Source: CAD feature listing. Evaluate the final solid. Frame: model axes, mm. A direction names the side the tool comes from. Coordinates: 2 decimals unless noted, no trailing zeros. Order: outer loops, then holes, each group sorted by start corner. A loop starts at its lowest first (then second) coordinate and runs counter-clockwise, first axis right, second up. Notation, with made-up numbers: (-39.5, 9.25) -> (-33.5, 9.25) arc R26 ccw to (-33.5, 38.25) -> close; hole circle Ø10 at (-40, 72.25). An arc over 180 degrees is marked (long way). Write item = value, one per line. Start each with the question number.
Item 1: Contact query for flat-ended pins moving along their axis: pin 1 (3.5 mm diameter, centred on x = 35, y = -50, fed in from +Z); pin 2 (1.9 mm diameter, centred on x = 50, y = 5, fed in from -Z). Output: stop coordinate, or through.
Item 2: Section query C-C (y = 0). Output: boundary loops of the cut face in (x, z).
Item 3: Section query A-A (y = -45). Output: boundary loops of the cut face in (x, z).
Item 4: Set-up query: faces 1 (the cylindrical face through (-51.526, 50.481, -6.549)), 2 (the cylindrical face through (-33.5, 27.117, -1.479)), 3 (the cylindrical face through (3.35, 47.85, -4.93)). Return all of +Z, -Z, +X, -X, +Y, -Y with unobstructed straight access to the full face (end or side cutting, diameter ignored); none if empty.
Item 5: Ray query, line 1 along Y through (x, z) = (35, -7.25); line 2 along X through (y, z) = (-4.5, -2); line 3 along X through (y, z) = (-44, -5.75). Return the intervals inside material, ascending. Write a range as [from, to].
Item 6: Section query D-D (x = 0.5). Output: boundary loops of the cut face in (y, z), then the cut area to 3 significant figures.
Item 7: Section query B-B (x = 45). Output: boundary loops of the cut face in (y, z).
```python
from build123d import *

# Parameters (mm, degrees)
F0_W           = 110
F0_H           = 110
F1_DEPTH       = 10
F2_D           = 3.2
F2_CBORE_D     = 6.5
F2_CBORE_DEPTH = 3
F3_D           = 4.2
F6_D           = 3.3
F6_DEPTH       = 14.1
F6_TIP         = 0.9914200214
F6_ON_F4_D     = 3.3
F6_ON_F4_DEPTH = 14.1
F6_ON_F4_TIP   = 0.9914200214
F7_D           = 5


with BuildPart() as f1:
    # F0 (on Top) → F1 (new body)
    with BuildSketch(Plane.XY):
        Rectangle(F0_W, F0_H)
    extrude(amount=-F1_DEPTH)

    # F2 (through all)
    with Locations(Plane.XY):
        with Locations((-50, 30), (-35, 30), (-35, 50), (-50, 50), (-50, -30), (-35, -30), (-35, -50), (-50, -50), (35, -30), (35, -50), (50, -50), (50, -30), (35, 30), (35, 50), (50, 50), (50, 30), (-50, 5), (-50, -5), (50, 5), (50, -5)):
            CounterBoreHole(F2_D / 2, F2_CBORE_D / 2, F2_CBORE_DEPTH)

    # F3 (through all)
    with Locations(Plane.XY):
        with Locations((-45, 45), (45, 45), (45, -45), (-45, -45)):
            Hole(F3_D / 2)

    # F6
    with Locations(Plane(origin=(0, 55, 0), x_dir=(-1, 0, 0), z_dir=(0, 1, 0))):
        with Locations((-5, -5), (5, -5)):
            Hole(F6_D / 2, depth=F6_DEPTH)
            with Locations((0, 0, -(F6_DEPTH + F6_TIP / 2))):  # 118° drill point
                Cone(0, F6_D / 2, F6_TIP, mode=Mode.SUBTRACT)

    # F6 on F4
    with Locations(Plane.XZ.offset(55)):
        with Locations((-5, -5), (5, -5)):
            Hole(F6_ON_F4_D / 2, depth=F6_ON_F4_DEPTH)
            with Locations((0, 0, -(F6_ON_F4_DEPTH + F6_ON_F4_TIP / 2))):  # 118° drill point
                Cone(0, F6_ON_F4_D / 2, F6_ON_F4_TIP, mode=Mode.SUBTRACT)

    # F7 (through all)
    with Locations(Plane.XY):
        with Locations((0, -45), (45, 0), (0, 45), (-45, 0)):
            Hole(F7_D / 2)


solid = f1.part
```
Computed:
q1.pin_1 = -3
q1.pin_2 = through
q2.outline = (-55, -10) -> (-47.5, -10) -> (-47.5, 0) -> (-55, 0) -> close; (-42.5, -10) -> (42.5, -10) -> (42.5, 0) -> (-42.5, 0) -> close; (47.5, -10) -> (55, -10) -> (55, 0) -> (47.5, 0) -> close
q3.outline = (-55, -10) -> (-47.1, -10) -> (-47.1, 0) -> (-55, 0) -> close; (-42.9, -10) -> (-2.5, -10) -> (-2.5, 0) -> (-42.9, 0) -> close; (2.5, -10) -> (42.9, -10) -> (42.9, 0) -> (2.5, 0) -> close; (47.1, -10) -> (55, -10) -> (55, 0) -> (47.1, 0) -> close; hole circle Ø3.3 at (-5, -5); hole circle Ø3.3 at (5, -5)
q4.face_1 = +Z, -Z
q4.face_2 = +Z
q4.face_3 = +Y
q5.line_1 = [-55, -51.6], [-48.4, -31.6], [-28.4, 28.4], [31.6, 48.4], [51.6, 55]
q5.line_2 = [-55, -53.21], [-46.79, 46.79], [53.21, 55]
q5.line_3 = [-55, -46.85], [-43.15, -6.47], [-3.53, -2.29], [2.29, 3.53], [6.47, 43.15], [46.85, 55]
q6.outline = (-55, -10) -> (-47.45, -10) -> (-47.45, 0) -> (-55, 0) -> close; (-42.55, -10) -> (42.55, -10) -> (42.55, 0) -> (-42.55, 0) -> close; (47.45, -10) -> (55, -10) -> (55, 0) -> (47.45, 0) -> close
q6.area = 1,000 mm^2
q7.outline = (-55, -10) -> (-47.1, -10) -> (-47.1, 0) -> (-55, 0) -> close; (-42.9, -10) -> (-2.5, -10) -> (-2.5, 0) -> (-42.9, 0) -> close; (2.5, -10) -> (42.9, -10) -> (42.9, 0) -> (2.5, 0) -> close; (47.1, -10) -> (55, -10) -> (55, 0) -> (47.1, 0) -> close
